```python
from build123d import *

# Parameters (mm, degrees)
F2_R     = 11.2
F3_DEPTH = 29.001


with BuildPart() as f1:
    # F0 (on Front) → F1 (revolve)
    with BuildSketch(Plane.XZ):
        Polygon((110.75, 45), (110.75, 0), (134.95, 0), (134.95, 2), (172.5, 2), (172.5, 29), (123, 29), (118.712813, 45), align=None)
    revolve(axis=Axis((0, 0, 22.5), (0, 0, 1)))

    # F2 (on face) → F3 (cut, through all)
    with BuildSketch(Plane.XY.offset(29)):
        with Locations((0, 149.25)):
            Circle(F2_R)
        with Locations((-105.535687, 105.535687)):
            Circle(F2_R)
        with Locations((-149.25, 0)):
            Circle(F2_R)
        with Locations((-105.535687, -105.535687)):
            Circle(F2_R)
        with Locations((0, -149.25)):
            Circle(F2_R)
        with Locations((105.535687, -105.535687)):
            Circle(F2_R)
        with Locations((149.25, 0)):
            Circle(F2_R)
        with Locations((105.535687, 105.535687)):
            Circle(F2_R)
    extrude(amount=-F3_DEPTH, mode=Mode.SUBTRACT)


solid = f1.part
```
Part model, mm, in its own coordinate system. A direction names the side the tool comes from. Round coordinates to 2 decimals unless told otherwise and drop trailing zeros. Loops run counter-clockwise (first coordinate to the right, second up) from the corner with the lowest first, then second, coordinate; pieces in that order, holes last. Notation, with made-up numbers: (-0.5, 54.25) -> (45.5, 54.25) arc R24 ccw to (45.5, 90.25) -> close; hole circle Ø11 at (5, 77). An arc over 180 degrees is marked (long way). Use one line per item in the form item = value. Start each with the question number.
Item 1: Two-plate mould, pull along X, no slides. Class faces 1 (the cylindrical face through (128.718, 40.535, 1.014)), 2 (the cylindrical face through (115.88, -109.83, 15.69)), 3 (the flat face through (11, 111, 0)): released by +X, released by -X, zero draft, split by the parting line, or undercut.
Item 2: Band-saw the part on A-A (y = 0). List the corners of the cut face in (x, z).
Item 3: Drill centre lines: line 1 along Y through (x, z) = (0, 13); line 2 along Y through (x, z) = (3.5, 9); line 3 along X through (y, z) = (78.5, 22). Where is each one in solid material? Low to high.
Item 4: Drop flat-ended pins along their axis: pin 1 Ø6 at (x, z) = (-80.5, 32.5) entering from -Y; pin 2 Ø8 at (x, y) = (109.5, 75.5) entering from +Z; pin 3 Ø12 at (y, z) = (-94, 17) entering from +X. Give the stop position or say it passes through.
Item 5: Tool access for faces 4 (the flat face through (-89, 103, 2)), 5 (the cylindrical face through (-160.44, 0.49, 15.69)), 6 (the flat face through (50, -114, 29)): list every direction of +Z, -Z, +X, -X, +Y, -Y with a clear straight run to the whole face (end or side of a thin tool).
Item 6: Band-saw the part on C-C (z = 6). Give the number of separate pieces and of enclosed holes in the cut face, plus the area to 3 significant figures.
Item 7: Band-saw the part on D-D (x = 149.25). List the corners of the cut face in (y, z), plus the area to 3 significant figures.
Data:
q1.face_1 = split by the parting line
q1.face_2 = undercut
q1.face_3 = zero draft
q2.outline = (-172.5, 2) -> (-160.45, 2) -> (-160.45, 29) -> (-172.5, 29) -> close; (-138.05, 2) -> (-134.95, 2) -> (-134.95, 0) -> (-110.75, 0) -> (-110.75, 45) -> (-118.71, 45) -> (-123, 29) -> (-138.05, 29) -> close; (110.75, 0) -> (134.95, 0) -> (134.95, 2) -> (138.05, 2) -> (138.05, 29) -> (123, 29) -> (118.71, 45) -> (110.75, 45) -> close; (160.45, 2) -> (172.5, 2) -> (172.5, 29) -> (160.45, 29) -> close
q3.line_1 = -172.5 to -160.45, -138.05 to -110.75, 110.75 to 138.05, 160.45 to 172.5
q3.line_2 = -172.46 to -159.89, -138.61 to -110.69, 110.69 to 138.61, 159.89 to 172.46
q3.line_3 = -153.6 to -78.12, 78.12 to 153.6
q4.pin_1 = -94.51
q4.pin_2 = 29
q4.pin_3 = 148.37
q5.face_4 = -Z
q5.face_5 = +Z, -Z
q5.face_6 = +Z
q6.separate_pieces = 1
q6.enclosed_holes = 9
q6.area = 51,800 mm^2
q7.outline = (-86.49, 2) -> (-11.2, 2) -> (-11.2, 29) -> (-86.49, 29) -> close; (11.2, 2) -> (86.49, 2) -> (86.49, 29) -> (11.2, 29) -> close
q7.area = 4,070 mm^2
